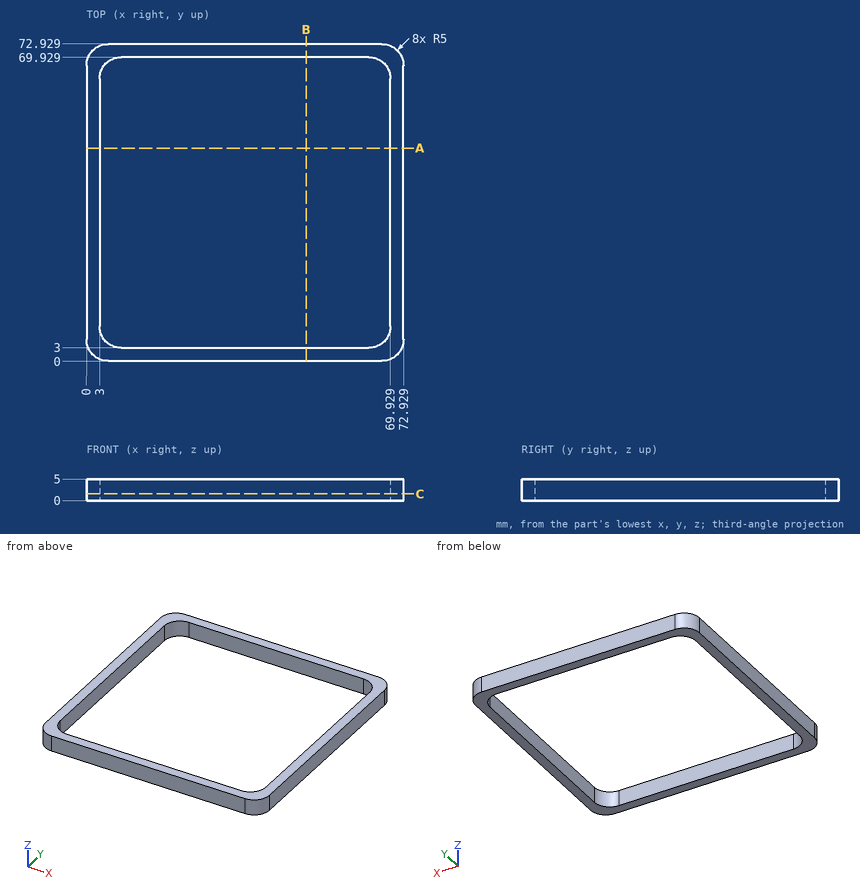
Design review of the part shown in the three views and the two pictorial views. Dimensions are in mm from the part's minimum x, y and z. Coordinates: 2 decimals unless noted, no trailing zeros. Loops run counter-clockwise (first coordinate to the right, second up) from the corner with the lowest first, then second, coordinate; pieces in that order, holes last. Notation, with made-up numbers: (7.25, 76.25) - (64.25, 76.25) arc R11 cw to (64.25, 83.25) - close; hole circle Ø5 at (37.5, -37.5). An arc over 180 degrees is marked (long way). Use a Markdown table: item, result. Add a question column.
Item 1: We need section C-C (z = 1.55). Give the boundary of the cut face in (x, y), and give its area (3 significant figures).
Item 2: We need section A-A (y = 49). Give the boundary of the cut face in (x, z), and give its area (3 significant figures).
Item 3: For line 1 (Y direction, x = 17.5, z = 3.9); line 2 (X direction, y = 68, z = 1.3), list the stretches that pass through material, from the lowest coordinate up.
Results list:
| question | item | result |
|---|---|---|
| 1 | outline | (0, 5) arc R5 ccw to (5, 0) - (67.93, 0) arc R5 ccw to (72.93, 5) - (72.93, 67.93) arc R5 ccw to (67.93, 72.93) - (5, 72.93) arc R5 ccw to (0, 67.93) - close; hole (3, 8) arc R5 ccw to (8, 3) - (64.93, 3) arc R5 ccw to (69.93, 8) - (69.93, 64.93) arc R5 ccw to (64.93, 69.93) - (8, 69.93) arc R5 ccw to (3, 64.93) - close |
| 1 | area | 839 mm^2 |
| 2 | outline | (0, 0) - (3, 0) - (3, 5) - (0, 5) - close; (69.93, 0) - (72.93, 0) - (72.93, 5) - (69.93, 5) - close |
| 2 | area | 30.0 mm^2 |
| 3 | line 1 | y = 0 to 3, 69.93 to 72.93 |
| 3 | line 2 | x = 0 to 4.05, 68.87 to 72.93 |
